Build history of the part. All positions in model axes, mm. Coordinates: 2 decimals unless noted, no trailing zeros. Loops run counter-clockwise (first coordinate to the right, second up) from the corner with the lowest first, then second, coordinate; pieces in that order, holes last. Notation, with made-up numbers: (40.5, 25.25) -> (50.5, 25.25) arc R27 ccw to (50.5, 58.25) -> close; hole circle Ø6 at (1, 6). An arc over 180 degrees is marked (long way). One line per item, written item: value. Start each with the question number.
```python
from build123d import *

# Parameters (mm, degrees)
SKETCH1_R      = 1.45
SKETCH1_R_2    = 1.44992108
SKETCH1_R_3    = 1
SKETCH1_R_4    = 1.5
SKETCH1_W      = 22.7
SKETCH1_H      = 12.5
SKETCH1_W_2    = 10
SKETCH1_H_2    = 2.952902408
SKETCH1_H_3    = 3.175
SKETCH1_W_3    = 3.175
SKETCH1_H_4    = 7
SKETCH1_W_4    = 28.701572838
SKETCH1_H_5    = 17.835977406
EXTRUDE1_DEPTH = 3.175


with BuildPart() as part:
    # Sketch1 → Extrude1 (new body)
    with BuildSketch(Plane(origin=(0, 0, 0), x_dir=(0, 0, -1), z_dir=(1, 0, 0))):
        Polygon((71.197724246, -30.438774567), (71.197724246, -37.036692127), (-106.598842421, -37.036692127), (-106.598842421, -30.436692127), (-96.598842421, -30.436692127), (-96.598842421, -27.261692127), (-106.598842421, -27.261692127), (-106.598842421, 2.738307873), (-96.598842421, 2.738307873), (-96.598842421, 5.913307873), (-106.598842421, 5.913307873), (-106.598842421, 15.913307873), (-38.865609087, 29.788307873), (-35.457953974, 29.936573589), (-35.457953974, 22.936573589), (-32.282953974, 22.936573589), (-32.282953974, 29.936573589), (-18.865609087, 29.788307873), (-18.865609087, -20.211692127), (71.197724246, -20.211692127), (71.197724246, -27.483789719), (61.197724246, -27.483789719), (61.197724246, -30.438774567), align=None)
        with Locations((-79.418842421, -28.849192127)):
            Circle(SKETCH1_R, mode=Mode.SUBTRACT)
        with Locations((6.481057579, -28.960240923)):
            Circle(SKETCH1_R_2, mode=Mode.SUBTRACT)
        with Locations((-60.661798953, -21.233789719)):
            Circle(SKETCH1_R_3, mode=Mode.SUBTRACT)
        with Locations((-32.961798953, -21.233789719)):
            Circle(SKETCH1_R_3, mode=Mode.SUBTRACT)
        with Locations((-33.870453974, 13.93657382)):
            Circle(SKETCH1_R, mode=Mode.SUBTRACT)
        with Locations((-74.848842421, 4.325807873)):
            Circle(SKETCH1_R_4, mode=Mode.SUBTRACT)
        with Locations((-46.811798953, -21.233789719)):
            Rectangle(SKETCH1_W, SKETCH1_H, mode=Mode.SUBTRACT)
        with Locations((-6.510665386, -28.960240923)):
            Rectangle(SKETCH1_W_2, SKETCH1_H_2, mode=Mode.SUBTRACT)
        with Locations((-48.098842421, 4.325807873)):
            Rectangle(SKETCH1_W_2, SKETCH1_H_3, mode=Mode.SUBTRACT)
        with Locations((-33.874298953, 1.43657382)):
            Rectangle(SKETCH1_W_3, SKETCH1_H_4, mode=Mode.SUBTRACT)
        with Locations((-83.72320649, -11.157017929)):
            Rectangle(SKETCH1_W_4, SKETCH1_H_5, mode=Mode.SUBTRACT)
    extrude(amount=EXTRUDE1_DEPTH)


solid = part.part
```
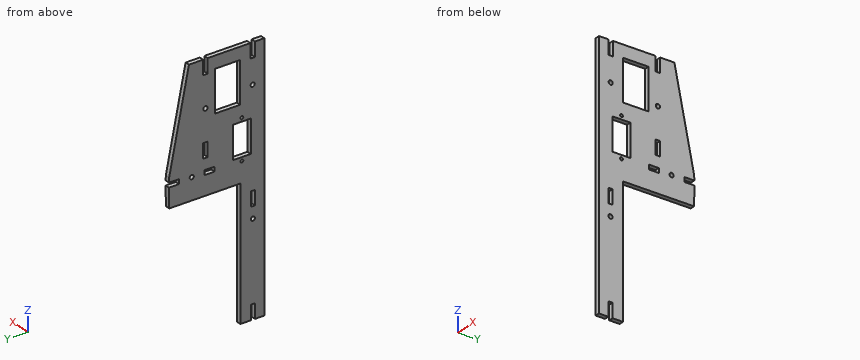
Item 1: Band-saw the part on A-A, the plane y = 1. List the corners of the cut face in (x, z) (3 decimals).
Item 2: Probe probe 1 along Z at (x, y) = (0.95, 4.5); probe 2 along Z at (x, y) = (1.5, -20); probe 3 along Y at (x, z) = (1.2, 7). List the from-to ranges inside material, lowest first.
Item 3: Band-saw the part on B-B, the plane z = 56. List the corners of the cut face in (x, y) (3 decimals), and give its area (3 significant figures).
Item 4: Band-saw the part on D-D, the plane z = -11. List the corners of the cut face in (x, y) (3 decimals).
Item 5: Band-saw the part on C-C, the plane x = 0.6. Count the separate pieces of the cut face and the enclosed holes in it, and give its area (3 significant figures).
Item 6: Drop flat-ended pins along their axis: pin 1 Ø1.6 at (x, z) = (1.5, 101.5) entering from +Y; pin 2 Ø1.6 at (x, z) = (1.5, -67.5) entering from +Y; pin 3 Ø5 at (y, z) = (-17, 12.5) entering from +X; pin 4 Ø1 at (x, z) = (2.5, 34.5) entering from +Y. Give the stop position or say it passes through.
Worked out:
1. outline: (0, 18.866) -> (3.175, 18.866) -> (3.175, 32.287) -> (0, 32.287) -> close; (0, 35.462) -> (3.175, 35.462) -> (3.175, 106.599) -> (0, 106.599) -> close
2. probe 1: z = 18.87 to 32.29, 35.46 to 43.1, 53.1 to 73.36, 76.34 to 96.6
2. probe 2: z = 18.87 to 35.46, 58.16 to 69.37, 98.07 to 106.6
2. probe 3: y = -37.04 to -30.44, -27.48 to -20.21
3. outline: (0, -37.037) -> (3.175, -37.037) -> (3.175, -27.484) -> (0, -27.484) -> close; (0, -14.984) -> (3.175, -14.984) -> (3.175, 26.278) -> (0, 26.278) -> close
3. area: 161 mm²
4. outline: (0, -37.037) -> (3.175, -37.037) -> (3.175, -20.212) -> (0, -20.212) -> close
5. separate pieces: 1
5. enclosed holes: 11
5. area: 5,880 mm²
6. pin 1: stops at y = 17.12
6. pin 2: stops at y = -20.21
6. pin 3: passes through
6. pin 4: stops at y = 22.94
